The drawing under review shows one solid part. Ordinate dimensions are in mm from its lowest x, y, z. A direction names the side the tool comes from. Coordinates: 2 decimals unless noted, no trailing zeros. Order: outer loops, then holes, each group sorted by start corner. A loop starts at its lowest first (then second) coordinate and runs counter-clockwise, first axis right, second up. Notation, with made-up numbers: (87, 29.5) - (109, 29.5) arc R29 cw to (109, 65.5) - close; hole circle Ø10 at (10, -2.75). An arc over 180 degrees is marked (long way). Answer in a Markdown table with one row per item.
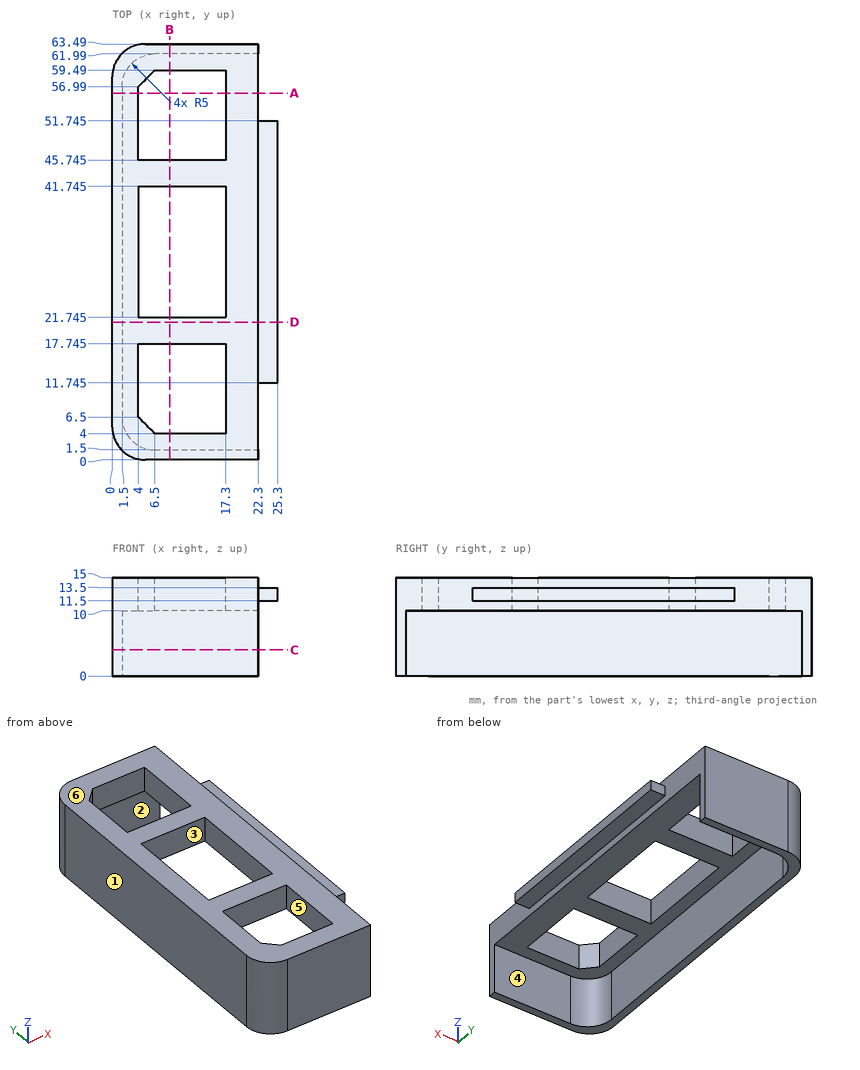
Item 1: We need section A-A, the plane y = 56. Write out the cut boundary in (x, z), then the cut area to 3 significant figures.
Check values:
| item | result |
|---|---|
| outline | (0, 0) - (1.5, 0) - (1.5, 10) - (4, 10) - (4, 15) - (0, 15) - close; (17.3, 10) - (22.3, 10) - (22.3, 15) - (17.3, 15) - close |
| area | 60.0 mm^2 |
Item 2: Mouldability with a two-part tool opening along X and no side actions: class the marked faces 1, 2 and 3 as +X half, -X half, draft (parallel to the pull), parting line (faces both ways), or undercut.
Check values:
| item | result |
|---|---|
| face 1 | -X half |
| face 2 | draft |
| face 3 | undercut |
Item 3: We need section C-C, the plane z = 4. Write out the cut boundary in (x, y), then the cut area to 3 significant figures.
Check values:
| item | result |
|---|---|
| outline | (0, 5) arc R5 ccw to (5, 0) - (22.3, 0) - (22.3, 1.5) - (6.5, 1.5) arc R5 cw to (1.5, 6.5) - (1.5, 56.99) arc R5 cw to (6.5, 61.99) - (22.3, 61.99) - (22.3, 63.49) - (5, 63.49) arc R5 ccw to (0, 58.49) - close |
| area | 158 mm^2 |
Item 4: We need section B-B, the plane x = 8.75. Write out the cut boundary in (y, z) (3 decimals).
Check values:
| item | result |
|---|---|
| outline | (0, 0) - (1.5, 0) - (1.5, 10) - (4, 10) - (4, 15) - (0, 15) - close; (17.745, 10) - (21.745, 10) - (21.745, 15) - (17.745, 15) - close; (41.745, 10) - (45.745, 10) - (45.745, 15) - (41.745, 15) - close; (59.49, 10) - (61.99, 10) - (61.99, 0) - (63.49, 0) - (63.49, 15) - (59.49, 15) - close |
Item 5: Tool access review of the marked faces 4, 5 and 6: name each direction out of +Z, -Z, +X, -X, +Y, -Y from which nothing blocks a thin tool from reaching the whole face with its end or side.
Check values:
| item | result |
|---|---|
| face 4 | -Z, +X |
| face 5 | +Z, -Z |
| face 6 | +Z, +X, -X, +Y, -Y |
Item 6: Clearance check with flat-ended pins moving along their axes: pin 1 Ø4 at (x, z) = (11.5, 12.5) entering from -Y; pin 2 Ø3 at (y, z) = (39, 4) entering from +X; pin 3 Ø0.6 at (x, z) = (24.5, 13) entering from +Y (3 decimals); pin 4 Ø0.6 at (x, z) = (24.5, 12.5) entering from -Y (3 decimals). State where each tip first meets the part, or that it passes through.
Check values:
| item | result |
|---|---|
| pin 1 | y = 0 |
| pin 2 | x = 1.5 |
| pin 3 | y = 51.745 |
| pin 4 | y = 11.745 |
Item 7: We need section D-D, the plane y = 21. Write out the cut boundary in (x, z).
Check values:
| item | result |
|---|---|
| outline | (0, 0) - (1.5, 0) - (1.5, 10) - (22.3, 10) - (22.3, 11.5) - (25.3, 11.5) - (25.3, 13.5) - (22.3, 13.5) - (22.3, 15) - (0, 15) - close |
Item 8: To check wall thickness, follow line 1 (Y direction, x = 13, z = 14) (3 decimals); line 2 (X direction, y = 57, z = 11.25); line 3 (Y direction, x = 6.25, z = 6.5). State the ranges of each line that lie inside material, in increasing order. Write a range as from..to.
Check values:
| item | result |
|---|---|
| line 1 | 0..4, 17.745..21.745, 41.745..45.745, 59.49..63.49 |
| line 2 | 0..4.01, 17.3..22.3 |
| line 3 | 0..1.51, 61.98..63.49 |
